Design review of the part built by this model. Coordinates are the model's own, in mm. A direction names the side the tool comes from. Round coordinates to 2 decimals unless told otherwise and drop trailing zeros. Order: outer loops, then holes, each group sorted by start corner. A loop starts at its lowest first (then second) coordinate and runs counter-clockwise, first axis right, second up. Notation, with made-up numbers: (39.25, 83) - (85.25, 83) arc R9 cw to (85.25, 98) - close; hole circle Ø6 at (-25.75, 65). An arc over 180 degrees is marked (long way). Write item = value, one per line.
from build123d import *

# Parameters (mm, degrees)
BOSS_EXTRUDE1_DEPTH = 40
SKETCH2_R           = 6.1
CUT_EXTRUDE1_DEPTH  = 40
CIRPATTERN1_COUNT   = 5
CIRPATTERN1_ANGLE   = 180
SKETCH3_R           = 6.1
CUT_EXTRUDE2_DEPTH  = 40
SKETCH5_R           = 50
CUT_EXTRUDE3_DEPTH  = 21
SKETCH6_R           = 42.5
CUT_EXTRUDE4_DEPTH  = 2
CHAMFER1_SIZE       = 2
FILLET1_R           = 3


with BuildPart() as part:
    # Sketch1 → Boss-Extrude1 (new body)
    with BuildSketch(Plane.XY):
        with BuildLine():
            Line((-81, 0), (-81, -150))
            Line((-81, -150), (81, -150))
            Line((81, -150), (81, 0))
            ThreePointArc((81, 0), (0, 81), (-81, 0))
        make_face()
    extrude(amount=BOSS_EXTRUDE1_DEPTH)

    # Sketch2 → Cut-Extrude1 (cut)
    with BuildSketch(Plane.XY.offset(40)):
        with Locations((-65, 0)):
            Circle(SKETCH2_R)
    cut_extrude1 = extrude(amount=-CUT_EXTRUDE1_DEPTH, mode=Mode.SUBTRACT)

    # CirPattern1: Cut-Extrude1 ×5 about axis
    cirpattern1_axis = Axis((0, 0, 0), (0, 0, -1))
    for i in range(1, CIRPATTERN1_COUNT):
        add(cut_extrude1.rotate(cirpattern1_axis, i * CIRPATTERN1_ANGLE / (CIRPATTERN1_COUNT - 1)), mode=Mode.SUBTRACT)

    # Sketch3 → Cut-Extrude2 (cut)
    with BuildSketch(Plane.XY.offset(40)):
        with Locations((-65, -135)):
            Circle(SKETCH3_R)
        with Locations((-65, -95)):
            Circle(SKETCH3_R)
        with Locations((-65, -55)):
            Circle(SKETCH3_R)
    cut_extrude2 = extrude(amount=-CUT_EXTRUDE2_DEPTH, mode=Mode.SUBTRACT)

    # Mirror1: Cut-Extrude2 across plane
    add(cut_extrude2.mirror(Plane(origin=(0, 0, 0), x_dir=(0, 0, 1), z_dir=(1, 0, 0))), mode=Mode.SUBTRACT)

    # Sketch5 → Cut-Extrude3 (cut)
    with BuildSketch(Plane.XY.offset(40)):
        Circle(SKETCH5_R)
    extrude(amount=-CUT_EXTRUDE3_DEPTH, mode=Mode.SUBTRACT)

    # Sketch6 → Cut-Extrude4 (cut)
    with BuildSketch(Plane.XY.offset(19)):
        Circle(SKETCH6_R)
    extrude(amount=-CUT_EXTRUDE4_DEPTH, mode=Mode.SUBTRACT)

    # Chamfer1
    chamfer1_edges = [part.edges().sort_by_distance(p)[0] for p in [
        (-50, 0, 40),
    ]]
    chamfer(chamfer1_edges, length=CHAMFER1_SIZE)

    # Fillet1
    fillet1_edges = [part.edges().sort_by_distance(p)[0] for p in [
        (81, -75, 0),
        (0, -150, 0),
        (-81, -75, 0),
        (0, 81, 0),
    ]]
    fillet(fillet1_edges, radius=FILLET1_R)


solid = part.part
1) We need section A-A on y = -135. Write out the cut boundary in (x, z), and give its area (3 significant figures).
Findings:
outline = (-81, 3) arc R3 ccw to (-78, 0) - (-71.1, 0) - (-71.1, 40) - (-81, 40) - close; (-58.9, 0) - (58.9, 0) - (58.9, 40) - (-58.9, 40) - close; (71.1, 0) - (78, 0) arc R3 ccw to (81, 3) - (81, 40) - (71.1, 40) - close
area = 5,500 mm^2
2) The part is to be moulded in two halves that separate along X. For faces 3 (the flat face through (-22, -37, 19)), 4 (the flat face through (81, -76, 21)), 5 (the flat face through (-81, -74, 21)), say which applies: released by +X, released by -X, zero draft, split by the parting line, or undercut.
Findings:
face_3 = undercut
face_4 = released by +X
face_5 = released by -X
3) We need section B-B on z = 22.5. Give the number of separate pieces and of enclosed holes in the cut face, and give its area (3 significant figures).
Findings:
separate_pieces = 1
enclosed_holes = 12
area = 25,500 mm^2
4) For faces 1 (the cylindrical face through (-66.322, -140.955, 20.28)), 2 (the cylindrical face through (-33.727, -25.861, 18.014)), list the 3-axis set-ups (+Z, -Z, +X, -X, +Y, -Y) from which the entire face can be reached by the end or side of a thin tool; tool diameter is ignored.
Findings:
face_1 = +Z, -Z
face_2 = +Z
5) Clearance check with flat-ended pins moving along their axes: pin 1 Ø6 at (x, y) = (-37.5, 5.5) entering from +Z; pin 2 Ø7.5 at (x, y) = (65, -95) entering from -Z; pin 3 Ø12 at (y, z) = (49, 5.5) entering from +X. State where each tip first meets the part, or that it passes through.
Findings:
pin_1 = 17
pin_2 = through
pin_3 = 68.64
6) To check wall thickness, follow L1, parallel to X at y = -5, z = 32.5; L2, parallel to Y at x = -64.5, z = 20; L3, parallel to X at y = -136, z = 32.5. State the ranges of each line that lie inside material, in increasing order. Write a range as from..to.
Findings:
L1 = -81..-68.49, -61.51..-49.75, 49.75..61.51, 68.49..81
L2 = -150..-141.08, -128.92..-101.08, -88.92..-61.08, -48.92..-6.08, 6.08..49
L3 = -81..-71.02, -58.98..58.98, 71.02..81
